Source: CAD feature listing. Evaluate the final solid. Frame: model axes, mm. A direction names the side the tool comes from. Give positions to 0.01 mm unless a question says otherwise; leave off trailing zeros. Write each loop counter-clockwise with the first axis right and the second up, starting at its lowest first coordinate (ties: lowest second). Pieces come first, ordered by that corner, then holes. Notation, with made-up numbers: (37, 26) -> (54, 26) arc R26 ccw to (54, 60) -> close; hole circle Ø6 at (70, 65.5). An arc over 180 degrees is marked (long way). Write item = value, one per line.
from build123d import *

# Parameters (mm, degrees)
SKETCH1_W                = 95
SKETCH1_H                = 42
BOSS_EXTRUDE2_DEPTH      = 2.5
EXTRUDE_THIN1_DEPTH      = 2.5
EXTRUDE_THIN1_DEPTH_BACK = 10
SKETCH1_2_W              = 100
SKETCH1_2_H              = 47
SKETCH1_2_W_2            = 95
SKETCH1_2_H_2            = 42
BOSS_EXTRUDE3_DEPTH      = 12.5
SKETCH2_4_W              = 55
SKETCH2_4_H              = 27.5
BOSS_EXTRUDE4_DEPTH      = 2.5


with BuildPart() as part:
    # Sketch1 → Boss-Extrude2 (new body)
    with BuildSketch(Plane(origin=(0, 0, 0), x_dir=(0, 0, -1), z_dir=(1, 0, 0))):
        with Locations((47.5, 21)):
            Rectangle(SKETCH1_W, SKETCH1_H)
    extrude(amount=BOSS_EXTRUDE2_DEPTH)

    # Sketch1<2> → Extrude-Thin1 (add, two sides: drawn at the far end of the back side and taken through both)
    with BuildSketch(Plane(origin=(0, 0, 0), x_dir=(0, 0, -1), z_dir=(1, 0, 0)).offset(-EXTRUDE_THIN1_DEPTH_BACK)):
        with Locations((47.5, 21)):
            Rectangle(SKETCH1_2_W, SKETCH1_2_H)
        with Locations((47.5, 21)):
            Rectangle(SKETCH1_2_W_2, SKETCH1_2_H_2, mode=Mode.SUBTRACT)
    extrude(amount=EXTRUDE_THIN1_DEPTH + EXTRUDE_THIN1_DEPTH_BACK)

    # Sketch2 → Boss-Extrude3 (add)
    with BuildSketch(Plane(origin=(2.5, 0, 0), x_dir=(0, 0, -1), z_dir=(1, 0, 0))):
        Polygon((95, 44.5), (97.5, 44.5), (97.5, 74.5), (40, 74.5), (40, 72), (95, 72), align=None)
    extrude(amount=-BOSS_EXTRUDE3_DEPTH)

    # Sketch2<4> → Boss-Extrude4 (add)
    with BuildSketch(Plane(origin=(2.5, 0, 0), x_dir=(0, 0, -1), z_dir=(1, 0, 0))):
        with Locations((67.5, 58.25)):
            Rectangle(SKETCH2_4_W, SKETCH2_4_H)
    extrude(amount=-BOSS_EXTRUDE4_DEPTH)


solid = part.part
(1) Section query C-C (y = 13.5). Return loops of the section in (x, z), plus the area to 3 significant figures.
Values follow:
outline = (-10, -97.5) -> (2.5, -97.5) -> (2.5, 2.5) -> (-10, 2.5) -> (-10, 0) -> (0, 0) -> (0, -95) -> (-10, -95) -> close
area = 300 mm2
(2) Access query for faces 5 (the face through (-4, 21, 2.5)), 6 (the face through (-5, 42, -47)), 7 (the face through (-5, 58, -95)). Directions: +Z, -Z, +X, -X, +Y, -Y. A direction counts if a zero-diameter tool reaches every point of the face in a straight line with its end or side. Return the directions, or none.
Values follow:
face_5 = +Z, +X, -X, +Y, -Y
face_6 = -X
face_7 = +Z, -X
(3) Pull-direction query (Z, two-part tool) for faces 1 (the face through (-4, 35, -97.5)), 2 (the face through (-5, 21, -95)), 3 (the face through (0.4, 62.8, -40)), 4 (the face through (0, 58, -67)); classes: pulls with the +Z half, pulls with the -Z half, needs draft (parallel to the pull), parting line crosses it, or undercut.
Values follow:
face_1 = pulls with the -Z half
face_2 = undercut
face_3 = pulls with the +Z half
face_4 = needs draft
(4) Section query A-A (x = -6). Return loops of the section in (y, z).
Values follow:
outline = (-2.5, -97.5) -> (74.5, -97.5) -> (74.5, -40) -> (72, -40) -> (72, -95) -> (44.5, -95) -> (44.5, 2.5) -> (-2.5, 2.5) -> close; hole (0, -95) -> (42, -95) -> (42, 0) -> (0, 0) -> close
(5) Material intervals for line 1 (Y direction, x = -1.25, z = -50); line 2 (Z direction, x = -6, y = 25.5); line 3 (Y direction, x = -2, z = -36.5), sorted ascending.
Values follow:
line_1 = -2.5 to 0, 42 to 44.5, 72 to 74.5
line_2 = -97.5 to -95, 0 to 2.5
line_3 = -2.5 to 0, 42 to 44.5
(6) Section query B-B (z = -31.5). Return loops of the section in (x, y), plus the area to 4 significant figures.
Values follow:
outline = (-10, -2.5) -> (2.5, -2.5) -> (2.5, 44.5) -> (-10, 44.5) -> (-10, 42) -> (0, 42) -> (0, 0) -> (-10, 0) -> close
area = 167.5 mm2
(7) Section query D-D (z = -77). Return loops of the section in (x, y).
Values follow:
outline = (-10, -2.5) -> (2.5, -2.5) -> (2.5, 74.5) -> (-10, 74.5) -> (-10, 72) -> (0, 72) -> (0, 44.5) -> (-10, 44.5) -> (-10, 42) -> (0, 42) -> (0, 0) -> (-10, 0) -> close
(8) First-contact query: pin 1 (6 mm diameter, centred on x = -1.5, y = 55.5, fed in from +Z). Flat tip, straight axial feed; report the tip coordinate or a pass-through.
Values follow:
pin_1 = -40
